Part model, mm, in its own coordinate system. Round coordinates to 2 decimals unless told otherwise and drop trailing zeros. Order: outer loops, then holes, each group sorted by start corner. A loop starts at its lowest first (then second) coordinate and runs counter-clockwise, first axis right, second up. Notation, with made-up numbers: (-14, 88) -> (37, 88) arc R21 cw to (37, 102) -> close; hole circle Ø9 at (21, -35.75). An arc over 180 degrees is marked (long way). Return JSON: item names as keys, results as strings. Group by question number.
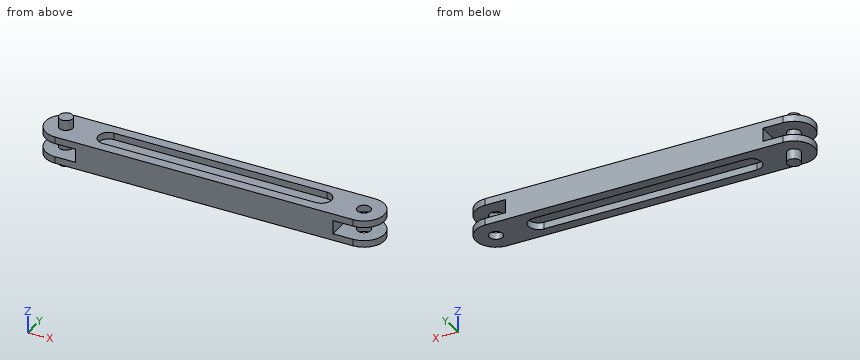
from build123d import *

# Parameters (mm, degrees)
SKETCH1_R                = 6.35
BOSS_EXTRUDE1_DEPTH      = 25.4
CUT_EXTRUDE1_DEPTH       = 6.35
SKETCH3_W                = 12.7
SKETCH3_H                = 38.1
CUT_EXTRUDE2_DEPTH       = 38.1
BOSS_EXTRUDE3_DEPTH      = 9.525
BOSS_EXTRUDE3_DEPTH_BACK = 34.925
SKETCH5_R                = 6.35


with BuildPart() as part:
    # Sketch1 → Boss-Extrude1 (new body)
    with BuildSketch(Plane.XY):
        with BuildLine():
            Line((0, 19.05), (280, 19.05))
            ThreePointArc((280, 19.05), (299.05, 0), (280, -19.05))
            Line((280, -19.05), (0, -19.05))
            ThreePointArc((0, -19.05), (-19.05, 0), (0, 19.05))
        make_face()
        Circle(SKETCH1_R, mode=Mode.SUBTRACT)
        with Locations((280, 0)):
            Circle(SKETCH1_R, mode=Mode.SUBTRACT)
    extrude(amount=BOSS_EXTRUDE1_DEPTH)

    # Sketch2 → Cut-Extrude1 (cut)
    with BuildSketch(Plane.XY.offset(25.4)):
        with BuildLine():
            Line((40, 9.525), (240, 9.525))
            ThreePointArc((240, 9.525), (249.525, 0), (240, -9.525))
            Line((240, -9.525), (40, -9.525))
            ThreePointArc((40, -9.525), (30.475, 0), (40, 9.525))
        make_face()
    cut_extrude1 = extrude(amount=-CUT_EXTRUDE1_DEPTH, mode=Mode.SUBTRACT)

    # Mirror1: Cut-Extrude1 across plane
    add(cut_extrude1.mirror(Plane.XY.offset(12.7)), mode=Mode.SUBTRACT)

    # Sketch3 → Cut-Extrude2 (cut)
    with BuildSketch(Plane.ZY.offset(19.05)):
        with Locations((12.7, 0)):
            Rectangle(SKETCH3_W, SKETCH3_H)
    cut_extrude2 = extrude(amount=-CUT_EXTRUDE2_DEPTH, mode=Mode.SUBTRACT)

    # Mirror2: Cut-Extrude2 across plane
    add(cut_extrude2.mirror(Plane.ZY.offset(-140)), mode=Mode.SUBTRACT)

    # Sketch5 → Boss-Extrude3 (add, two sides: drawn at the far end of the back side and taken through both)
    with BuildSketch(Plane.XY.offset(25.4).offset(-BOSS_EXTRUDE3_DEPTH_BACK)):
        Circle(SKETCH5_R)
    extrude(amount=BOSS_EXTRUDE3_DEPTH + BOSS_EXTRUDE3_DEPTH_BACK)


solid = part.part
(1) Pin check, flat tips, straight feed: P1, Ø5, axis at y = 13, z = -2, coming from the -X side; P2, Ø12, axis at x = 52.5, y = 12, coming from the -Z side; P3, Ø9.5, axis at x = 135, y = 4.5, coming from the +Z side. Stop position of each tip, or through.
(2) Saw through at C-C, the plane z = 29. List the corners of the cut face in (x, y).
(3) Saw through at B-B, the plane x = 80.5. List the corners of the cut face in (y, z) (3 decimals).
(4) Saw through at A-A, the plane z = 10. List the corners of the cut face in (x, y).
(5) Probe L1, parallel to X at y = 0, z = 24 (3 decimals); L2, parallel to Z at x = 280, y = 8; L3, parallel to Y at x = 280, z = 3. List the from-to ranges inside material, lowest first. Write a range as [from, to].
Results are:
{
 "1": {"P1": "stops at x = -15.19", "P2": "stops at z = 0", "P3": "stops at z = 19.05"},
 "2": {"outline": "circle Ø12.7 at (0, 0)"},
 "3": {"outline": "(-19.05, 0) -> (-9.525, 0) -> (-9.525, 6.35) -> (9.525, 6.35) -> (9.525, 0) -> (19.05, 0) -> (19.05, 25.4) -> (9.525, 25.4) -> (9.525, 19.05) -> (-9.525, 19.05) -> (-9.525, 25.4) -> (-19.05, 25.4) -> close"},
 "4": {"outline": "circle Ø12.7 at (0, 0); (19.05, -19.05) -> (260.95, -19.05) -> (260.95, 19.05) -> (19.05, 19.05) -> close"},
 "5": {"L1": "x = [-19.05, 30.475], [249.525, 273.65], [286.35, 299.05]", "L2": "z = [0, 6.35], [19.05, 25.4]", "L3": "y = [-19.05, -6.35], [6.35, 19.05]"}
}
